Here's how the part is built. I have some questions about the finished solid (model axes, mm). Face numbers are marked on the shaded views. A direction names the side the tool comes from. Round coordinates to 2 decimals unless told otherwise and drop trailing zeros. Order: outer loops, then holes, each group sorted by start corner. A loop starts at its lowest first (then second) coordinate and runs counter-clockwise, first axis right, second up. Notation, with made-up numbers: (14.25, -40) - (64.25, -40) arc R16 ccw to (64.25, -32) - close; hole circle Ø7 at (46.25, 41). An arc over 180 degrees is marked (long way). One line per item, written item: value.
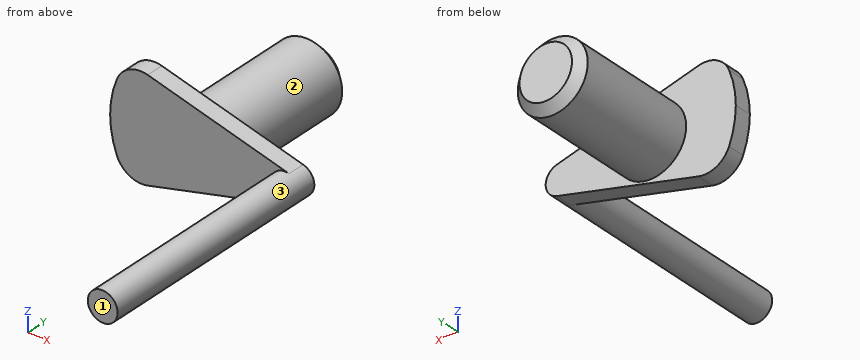
from build123d import *

# Parameters (mm, degrees)
F1_DEPTH = 2
F3_DEPTH = 26
F4_R     = 4
F5_DEPTH = 15
F6_SIZE  = 1


with BuildPart() as f1:
    # F0 (on Front) → F1 (new body)
    with BuildSketch(Plane.XZ):
        with BuildLine():
            ThreePointArc((10.7772780728, -1.6469869803), (11.6988240407, -1.0425715004), (12.0560490534, 0))
            ThreePointArc((12.0560490534, 0), (11.6988240407, 1.0425715004), (10.7772780728, 1.6469869803))
            Line((10.7772780728, 1.6469869803), (-5.3807416604, 5.7795192287))
            ThreePointArc((-5.3807416604, 5.7795192287), (-7.4835794739, 5.5473528625), (-8.9103223258, 3.9852283712))
            ThreePointArc((-8.9103223258, 3.9852283712), (-9.4830781383, 2.0290875977), (-9.6763123684, 0))
            ThreePointArc((-9.6763123684, 0), (-9.4830781383, -2.0290875977), (-8.9103223258, -3.9852283712))
            ThreePointArc((-8.9103223258, -3.9852283712), (-7.4835794739, -5.5473528625), (-5.3807416604, -5.7795192287))
            Line((-5.3807416604, -5.7795192287), (10.7772780728, -1.6469869803))
        make_face()
    extrude(amount=F1_DEPTH)

    # F2 (on face) → F3 (join)
    with BuildSketch(Plane.XZ.offset(2)):
        with BuildLine():
            ThreePointArc((10.7772780728, -1.6469869803), (11.6988240407, -1.0425715004), (12.0560490534, 0))
            ThreePointArc((12.0560490534, 0), (11.6988240407, 1.0425715004), (10.7772780728, 1.6469869803))
            ThreePointArc((10.7772780728, 1.6469869803), (8.6560490534, 0), (10.7772780728, -1.6469869803))
        make_face()
    extrude(amount=F3_DEPTH)

    # F4 (on face) → F5 (join)
    with BuildSketch(Plane(origin=(0, 0, 0), x_dir=(-1, 0, 0), z_dir=(0, 1, 0))):
        Circle(F4_R)
    extrude(amount=F5_DEPTH)

    # F6
    f6_edges = [f1.edges().sort_by_distance(p)[0] for p in [
        (4, 15, 0),
    ]]
    chamfer(f6_edges, length=F6_SIZE)


solid = f1.part
Q1. If we section it at B-B, the plane y = 2: Please give me the cut outline in (x, z), then the cut area to 3 significant figures.
Results list:
outline: circle Ø8 at (0, 0)
area: 50.3 mm²
Q2. Will these pins go through, and if not, where does the flat tip stop? pin 1 (1.5 mm diameter, centred on y = 5.5, z = 0.5, fed in from +X); pin 2 (1.5 mm diameter, centred on x = 2.5, z = -2, fed in from -Y); pin 3 (12 mm diameter, centred on x = 8.5, y = 2.5, fed in from +Z).
Results list:
pin 1: x = 4
pin 2: y = -2
pin 3: z = 3.62
Q3. Which directions (+Z, -Z, +X, -X, +Y, -Y) give clear straight access to the entire face, cutting with the end or side of a thin tool? Please do the marked faces 1, 2 and 3.
Results list:
face 1: +Z, -Z, +X, -X, -Y
face 2: +Y
face 3: -Y
Q4. If we section it at D-D, the plane x = 7.5: Please give me the cut outline in (y, z), then the cut area to 3 significant figures.
Results list:
outline: (-2, -2.49) - (0, -2.49) - (0, 2.49) - (-2, 2.49) - close
area: 9.94 mm²
Q5. If we section it at A-A, the plane x = 0: Please give me the cut outline in (y, z), then the cut area to 3 significant figures.
Results list:
outline: (-2, -4.4) - (0, -4.4) - (0, -4) - (14, -4) - (15, -3) - (15, 3) - (14, 4) - (0, 4) - (0, 4.4) - (-2, 4.4) - close
area: 137 mm²
Q6. If we section it at C-C, the plane y = -23.5: Please give me the cut outline in (x, z).
Results list:
outline: circle Ø3.4 at (10.36, 0)
Q7. If I drill on line 1 along Y through (x, z) = (-2.25, 1.5); line 2 along Y through (x, z) = (-8.5, 2.5); line 3 along Z through (x, y) = (2.75, 13), over which ranges is the centre line in solid material (lowest first)?
Results list:
line 1: -2 to 15
line 2: -2 to 0
line 3: -2.9 to 2.9
